from build123d import *

# Parameters (mm, degrees)
SKETCH1_W                = 165.1
SKETCH1_H                = 76.2
BOSS_EXTRUDE1_DEPTH      = 6.35
M5_CLEARANCE_HOLE1_D     = 5.5
M5_CLEARANCE_HOLE1_DEPTH = 12.7
M5_CLEARANCE_HOLE1_TIP   = 1.652366702
SKETCH5_R                = 8
CUT_EXTRUDE1_DEPTH       = 6.35
FILLET1_R                = 6.35


with BuildPart() as part:
    # Sketch1 → Boss-Extrude1 (new body)
    with BuildSketch(Plane(origin=(0, 0, 0), x_dir=(1, 0, 0), z_dir=(0, 1, 0))):
        Rectangle(SKETCH1_W, SKETCH1_H)
    extrude(amount=BOSS_EXTRUDE1_DEPTH)

    # M5 Clearance Hole1
    with Locations(Plane(origin=(0, 6.35, 0), x_dir=(1, 0, 0), z_dir=(0, 1, 0))):
        with Locations((-44.45, 10), (-44.45, -10), (-18.45, 0), (-10.45, 23.999999994), (-10.45, -24.000000006), (-30.45, 23.999999994), (-30.45, -24.000000006)):
            Hole(M5_CLEARANCE_HOLE1_D / 2, depth=M5_CLEARANCE_HOLE1_DEPTH)
            with Locations((0, 0, -(M5_CLEARANCE_HOLE1_DEPTH + M5_CLEARANCE_HOLE1_TIP / 2))):  # 118° drill point
                Cone(0, M5_CLEARANCE_HOLE1_D / 2, M5_CLEARANCE_HOLE1_TIP, mode=Mode.SUBTRACT)

    # Sketch5 → Cut-Extrude1 (cut)
    with BuildSketch(Plane(origin=(0, 6.35, 0), x_dir=(1, 0, 0), z_dir=(0, 1, 0))):
        with Locations(Location((-18.45, 0, 0), (0, 0, 270))):
            Circle(SKETCH5_R)
    extrude(amount=-CUT_EXTRUDE1_DEPTH, mode=Mode.SUBTRACT)

    # Fillet1
    fillet1_edges = [part.edges().sort_by_distance(p)[0] for p in [
        (82.55, 3.175, 38.1),
        (-82.55, 3.175, 38.1),
        (-82.55, 3.175, -38.1),
        (82.55, 3.175, -38.1),
    ]]
    fillet(fillet1_edges, radius=FILLET1_R)


solid = part.part
The listing builds one solid part. Answer for the finished solid, in the listing's coordinates (mm). Coordinates: 2 decimals unless noted, no trailing zeros. Order: outer loops, then holes, each group sorted by start corner. A loop starts at its lowest first (then second) coordinate and runs counter-clockwise, first axis right, second up. Notation, with made-up numbers: (-28.75, -13.5) -> (13.25, -13.5) arc R28 cw to (13.25, 10.5) -> close; hole circle Ø10 at (77, 2). An arc over 180 degrees is marked (long way). Answer in a Markdown table with one row per item. Add a question column.
Item 1: Find section C-C (z = 24). Write down the section's boundary in (x, y).
Item 2: Find section A-A (z = 0). Write down the section's boundary in (x, y), then the cut area to 3 significant figures.
Item 3: Find section B-B (x = -44.45). Write down the section's boundary in (y, z), then the cut area to 3 significant figures.
Item 4: Find section D-D (y = 2). Write down the section's boundary in (x, z).
Item 5: This flat-tipped pin is pushed along its axis until it touches: P1, Ø5, axis at x = -10.45, z = 24, coming from the +Y side. Where does it stop, or does it pass through?
Item 6: Find the intervals of material crossed by L1, parallel to Z at x = -30.45, y = 2; L2, parallel to Z at x = -44.45, y = 5.25; L3, parallel to X at y = 1.75, z = 2, in increasing order. Write a range as from..to.
Item 7: Determine the mould class of faces 1 (the face through (-1, 0, -1)), 2 (the face through (-1, 3, 38.1)), 3 (the face through (-10.092, 3.131, -26.727)), 4 (the face through (-80.74, 3.22, -36.19)) for opening direction Z: +Z half, -Z half, draft (parallel to the pull), parting line (faces both ways), or undercut.
Result set:
| question | item | result |
|---|---|---|
| 1 | outline | (-82.55, 0) -> (-33.2, 0) -> (-33.2, 6.35) -> (-82.55, 6.35) -> close; (-27.7, 0) -> (-13.2, 0) -> (-13.2, 6.35) -> (-27.7, 6.35) -> close; (-7.7, 0) -> (82.55, 0) -> (82.55, 6.35) -> (-7.7, 6.35) -> close |
| 2 | outline | (-82.55, 0) -> (-26.45, 0) -> (-26.45, 6.35) -> (-82.55, 6.35) -> close; (-10.45, 0) -> (82.55, 0) -> (82.55, 6.35) -> (-10.45, 6.35) -> close |
| 2 | area | 947 mm² |
| 3 | outline | (0, -38.1) -> (6.35, -38.1) -> (6.35, -12.75) -> (0, -12.75) -> close; (0, -7.25) -> (6.35, -7.25) -> (6.35, 7.25) -> (0, 7.25) -> close; (0, 12.75) -> (6.35, 12.75) -> (6.35, 38.1) -> (0, 38.1) -> close |
| 3 | area | 414 mm² |
| 4 | outline | (-82.55, -31.75) arc R6.35 ccw to (-76.2, -38.1) -> (76.2, -38.1) arc R6.35 ccw to (82.55, -31.75) -> (82.55, 31.75) arc R6.35 ccw to (76.2, 38.1) -> (-76.2, 38.1) arc R6.35 ccw to (-82.55, 31.75) -> close; hole circle Ø5.5 at (-44.45, -10); hole circle Ø5.5 at (-44.45, 10); hole circle Ø5.5 at (-30.45, -24); hole circle Ø5.5 at (-30.45, 24); hole circle Ø16 at (-18.45, 0); hole circle Ø5.5 at (-10.45, -24); hole circle Ø5.5 at (-10.45, 24) |
| 5 | P1 | passes through |
| 6 | L1 | z = -38.1..-26.75, -21.25..21.25, 26.75..38.1 |
| 6 | L2 | z = -38.1..-12.75, -7.25..7.25, 12.75..38.1 |
| 6 | L3 | x = -82.55..-26.2, -10.7..82.55 |
| 7 | face 1 | draft |
| 7 | face 2 | +Z half |
| 7 | face 3 | undercut |
| 7 | face 4 | -Z half |
